```python
from build123d import *

# Parameters (mm, degrees)
F1_DEPTH  = 15.81
F2_R      = 2.455
F3_DEPTH  = 2
F4_W      = 6.363237
F4_H      = 12.76
F5_DEPTH  = 10
F6_W      = 8
F6_H      = 12.760826
F7_DEPTH  = 10
F9_DEPTH  = 15.84
F10_R     = 3.245
F10_R_2   = 2.425
F11_DEPTH = 9


with BuildPart() as f1:
    # F0 (on Front) → F1 (new body)
    with BuildSketch(Plane.XZ):
        Polygon((-2.968959, 0.465274), (-10.908959, 0.465274), (-10.908959, -9.104726), (5.051041, -9.104726), align=None)
    extrude(amount=F1_DEPTH)

    # F2 (on Top) → F3 (join)
    with BuildSketch(Plane.XY):
        with Locations((-6.943959, -3.975)):
            Circle(F2_R)
        with Locations((-6.943959, -11.955)):
            Circle(F2_R)
    extrude(amount=F3_DEPTH)

    # F4 (on Top) → F5 (cut)
    with BuildSketch(Plane.XY):
        with Locations((-6.197341, -7.9)):
            Rectangle(F4_W, F4_H)
    extrude(amount=-F5_DEPTH, mode=Mode.SUBTRACT)

    # F6 (on Top) → F7 (cut)
    with BuildSketch(Plane.XY):
        with Locations((-0.388959, -7.919587)):
            Rectangle(F6_W, F6_H)
    extrude(amount=-F7_DEPTH, mode=Mode.SUBTRACT)

    # F8 (on Front) → F9 (join)
    with BuildSketch(Plane.XZ):
        Polygon((4.992922, -8.935911), (-2.972763, 0.511219), (-4.48452, 0.511219), (2.988079, -8.935911), align=None)
    extrude(amount=F9_DEPTH)

    # F10 (on Top) → F11 (join)
    with BuildSketch(Plane.XY):
        with Locations((-2.943959, -8.171717)):
            Circle(F10_R)
        with Locations((-2.943959, -8.171717)):
            Circle(F10_R_2, mode=Mode.SUBTRACT)
    extrude(amount=-F11_DEPTH)


solid = f1.part
```
The listing builds one solid part. Answer for the finished solid, in the listing's coordinates (mm). A direction names the side the tool comes from. Coordinates: 2 decimals unless noted, no trailing zeros. Loops run counter-clockwise (first coordinate to the right, second up) from the corner with the lowest first, then second, coordinate; pieces in that order, holes last. Notation, with made-up numbers: (10, 60) -> (67, 60) arc R22 cw to (67, 97) -> close; hole circle Ø11 at (56, 17). An arc over 180 degrees is marked (long way). Use one line per item in the form item = value. Start each with the question number.
Item 1: Consider L1, parallel to X at y = -6.5, z = -8; L2, parallel to X at y = -7.75, z = -3.25; L3, parallel to Y at x = -8.5, z = -0.75. Determine where each line is inside the solid, lowest interval first. Write a range as [from, to].
Item 2: Flat-ended cylindrical pins translate along their axes: pin 1 Ø1.9 at (x, z) = (-6.5, -4.5) entering from -Y; pin 2 Ø4.5 at (y, z) = (-6.5, -4) entering from +X; pin 3 Ø1.7 at (x, y) = (-4, -7.5) entering from +Z. Find the tip coordinate at first contact, or state that the pin passes through.
Item 3: The part is cut by section A-A on z = -3.75. Determine the outline of the cut face in (x, y) (3 decimals).
Item 4: A tool of negligible diameter and unlimited length cuts with its end or side. For faces 1 (the face through (-4, -8, 0.511)), 2 (the face through (-5, -15.81, -5)), 3 (the face through (-5, -8, 0)), from which of +Z, -Z, +X, -X, +Y, -Y can it reach the whole face along a straight path? Write none if from no direction.
Item 5: The part is cut by section D-D on x = -7.5. Determine the outline of the cut face in (y, z), then the cut area to 3 significant figures.
Item 6: The part is cut by section B-B on y = -4.25. Determine the outline of the cut face in (x, z), then the cut area to 3 significant figures.
Item 7: The mould has two halves that part along X. Classify faces 4 (the face through (0.19, -6.4, -5.4)), 5 (the face through (-7, -14.28, -4)), 6 (the face through (-3, -15, -9.105)), 7 (the face through (0.3, -8.2, -1.3)): released by +X, released by -X, zero draft, split by the parting line, or undercut.
Item 8: The part is cut by section C-C on z = -1. Determine the outline of the cut face in (x, y) (3 decimals).
Answer key:
q1.L1 = [-10.91, -9.38], [-5.73, -4.7], [-1.19, -0.16], [2.25, 4.2]
q1.L2 = [-10.91, -9.38], [-6.16, -5.33], [-1.51, 0.27]
q1.L3 = [-15.81, -14.28], [-1.52, 0]
q2.pin_1 = -15.81
q2.pin_2 = 2.73
q2.pin_3 = 0.51
q3.outline = (-10.909, -15.81) -> (-1.114, -15.81) -> (-1.114, -15.84) -> (0.62, -15.84) -> (0.62, 0) -> (-10.909, 0) -> close; hole (-9.379, -14.28) -> (-4.389, -14.28) -> (-4.389, -14.3) -> (-1.114, -14.3) -> (-1.114, -10.851) arc R3.245 cw (long way) to (-1.114, -5.492) -> (-1.114, -1.539) -> (-3.016, -1.539) -> (-3.016, -1.52) -> (-9.379, -1.52) -> close; hole (-1.114, -9.763) -> (-1.114, -6.581) arc R2.425 ccw (long way) to start
q4.face_1 = +Z, +X, +Y, -Y
q4.face_2 = -Z, -X, -Y
q4.face_3 = -Z
q5.outline = (-15.81, -9.1) -> (-14.28, -9.1) -> (-14.28, 0) -> (-1.52, 0) -> (-1.52, -9.1) -> (0, -9.1) -> (0, 0.47) -> (-1.58, 0.47) -> (-1.58, 2) -> (-6.37, 2) -> (-6.37, 0.47) -> (-9.56, 0.47) -> (-9.56, 2) -> (-14.35, 2) -> (-14.35, 0.47) -> (-15.81, 0.47) -> close
q5.area = 49.8 mm2
q6.outline = (-10.91, -9.1) -> (-9.38, -9.1) -> (-9.38, 0) -> (-4.08, 0) -> (2.99, -8.94) -> (3.61, -8.94) -> (3.61, -9.1) -> (5.05, -9.1) -> (4.91, -8.94) -> (4.99, -8.94) -> (-2.97, 0.51) -> (-4.48, 0.51) -> (-4.45, 0.47) -> (-4.5, 0.47) -> (-4.5, 2) -> (-9.38, 2) -> (-9.38, 0.47) -> (-10.91, 0.47) -> close
q6.area = 41.4 mm2
q7.face_4 = undercut
q7.face_5 = undercut
q7.face_6 = zero draft
q7.face_7 = released by +X
q8.outline = (-10.909, -15.81) -> (-3.289, -15.81) -> (-3.289, -15.84) -> (-1.699, -15.84) -> (-1.699, -11.168) arc R3.245 ccw to (-1.699, -5.175) -> (-1.699, 0) -> (-10.909, 0) -> close; hole (-9.379, -14.28) -> (-4.389, -14.28) -> (-4.389, -14.3) -> (-3.289, -14.3) -> (-3.289, -11.398) arc R3.245 cw to (-3.289, -4.945) -> (-3.289, -1.52) -> (-9.379, -1.52) -> close; hole (-3.289, -10.572) -> (-3.289, -5.771) arc R2.425 ccw to start; hole (-1.699, -10.252) arc R2.425 ccw to (-1.699, -6.091) -> close
